Could you check a few things on this model? Use its own coordinates, in mm. Face numbers are marked on the shaded views. A direction names the side the tool comes from. Give positions to 0.01 mm unless a question says otherwise; leave off trailing zeros. Loops run counter-clockwise (first coordinate to the right, second up) from the corner with the lowest first, then second, coordinate; pieces in that order, holes last. Notation, with made-up numbers: (51, -2) - (80, -2) arc R28 cw to (80, 27) - close; hole circle Ø5 at (43, -28). An arc over 180 degrees is marked (long way). Write each question's results on one line, items separated by ' | '. Start each with the question number.
1) If we mould it in two halves opening along X, with no side actions, what happens to the marked faces 3, 4 and 5? For each: +X half, -X half, draft (parallel to the pull), parting line (faces both ways), or undercut.
2) If I drill on probe 1 along X at (y, z) = (2.95, -2.5); probe 2 along Z at (x, y) = (-1.25, 3.05); probe 3 along Z at (x, y) = (-0.25, 2.45), over which ranges is the centre line in solid material (lowest first)? Write a range as [from, to].
3) I'm going to push a flat-ended pin straight in: pin 1 (1 mm diameter, centred on x = -1, z = 2, fed in from -Y). Where does the tip first touch, or does it pass through?
4) On a 3-axis mill with a long thin cutter (end or side, diameter ignored), from which of +Z, -Z, +X, -X, +Y, -Y can I reach the whole of each face in a straight line? I mean the marked faces 1 and 2. Say none if no direction works.
5) I want a section at A-A, the plane z = 0.25. Write out the boundary of the cut face in (x, y).
6) I want a section at D-D, the plane x = 1.5. Write out the boundary of the cut face in (y, z), and give its area (3 significant figures).
7) I want a section at B-B, the plane x = 0. Write out the boundary of the cut face in (y, z), and give its area (3 significant figures).
8) I want a section at C-C, the plane y = 3.15. Write out the boundary of the cut face in (x, z), and give its area (3 significant figures).
from build123d import *

# Parameters (mm, degrees)
SKETCH1_W           = 6.8
SKETCH1_H           = 14.5
SKETCH1_W_2         = 4.8
SKETCH1_H_2         = 12.5
BOSS_EXTRUDE1_DEPTH = 3.5
BOSS_EXTRUDE2_DEPTH = 3.5


with BuildPart() as part:
    # Sketch1 → Boss-Extrude1 (new body)
    with BuildSketch(Plane(origin=(0, 0, 0), x_dir=(1, 0, 0), z_dir=(0, 1, 0))):
        Rectangle(SKETCH1_W, SKETCH1_H)
        Rectangle(SKETCH1_W_2, SKETCH1_H_2, mode=Mode.SUBTRACT)
    extrude(amount=BOSS_EXTRUDE1_DEPTH)

    # Sketch2 → Boss-Extrude2 (add)
    with BuildSketch(Plane(origin=(0, 3.5, 0), x_dir=(1, 0, 0), z_dir=(0, 1, 0))):
        with BuildLine():
            Line((-3.4, 7.25), (3.4, 7.25))
            Line((3.4, 7.25), (3.4, 8.25))
            ThreePointArc((3.4, 8.25), (0, 11.65), (-3.4, 8.25))
            Line((-3.4, 8.25), (-3.4, 7.25))
        make_face()
        with BuildLine():
            Line((-2.4, 8.25), (2.4, 8.25))
            ThreePointArc((2.4, 8.25), (0, 10.65), (-2.4, 8.25))
        make_face(mode=Mode.SUBTRACT)
    extrude(amount=-BOSS_EXTRUDE2_DEPTH)


solid = part.part
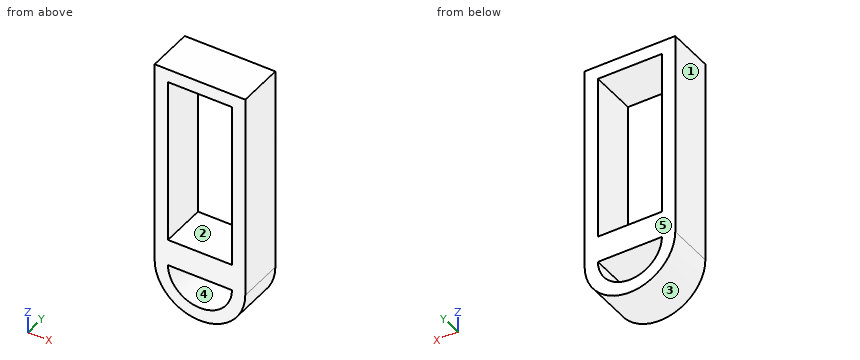
Answers:
1) face 3: parting line | face 4: undercut | face 5: draft
2) probe 1: x = [-3.4, -2.4], [2.4, 3.4] | probe 2: z = [-11.41, -10.3], [-8.25, -6.25], [6.25, 7.25] | probe 3: z = [-11.64, -10.64], [-8.25, -6.25], [6.25, 7.25]
3) pin 1: passes through
4) face 1: +Z, -Z, -X, +Y, -Y | face 2: +Y, -Y
5) outline: (-3.4, 0) - (-2.4, 0) - (-2.4, 3.5) - (-3.4, 3.5) - close; (2.4, 0) - (3.4, 0) - (3.4, 3.5) - (2.4, 3.5) - close
6) outline: (0, -11.3) - (3.5, -11.3) - (3.5, -10.12) - (0, -10.12) - close; (0, -8.25) - (3.5, -8.25) - (3.5, -6.25) - (0, -6.25) - close; (0, 6.25) - (3.5, 6.25) - (3.5, 7.25) - (0, 7.25) - close | area: 14.6 mm2
7) outline: (0, -11.65) - (3.5, -11.65) - (3.5, -10.65) - (0, -10.65) - close; (0, -8.25) - (3.5, -8.25) - (3.5, -6.25) - (0, -6.25) - close; (0, 6.25) - (3.5, 6.25) - (3.5, 7.25) - (0, 7.25) - close | area: 14.0 mm2
8) outline: (-3.4, -8.25) arc R3.4 ccw to (3.4, -8.25) - (3.4, 7.25) - (-3.4, 7.25) - close; hole (-2.4, -8.25) arc R2.4 ccw to (2.4, -8.25) - close; hole (-2.4, -6.25) - (2.4, -6.25) - (2.4, 6.25) - (-2.4, 6.25) - close | area: 54.5 mm2
